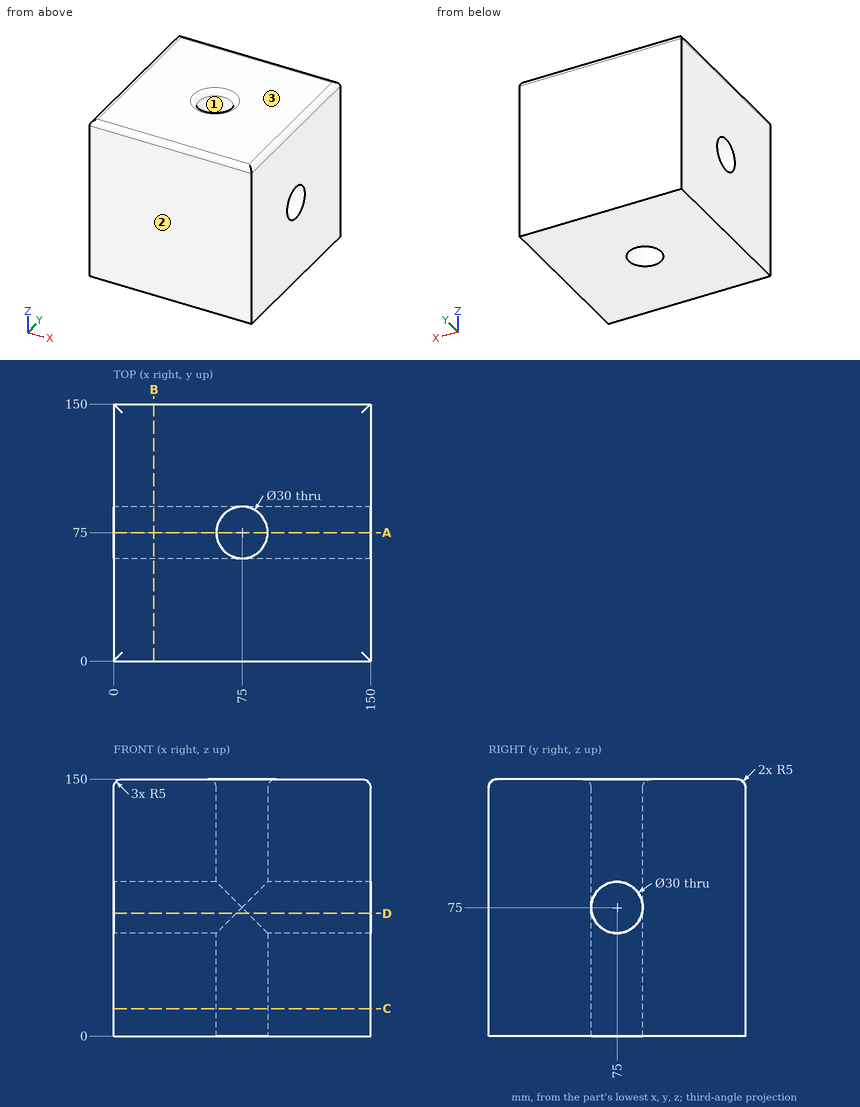
Here's the drawing with two shaded views (mm, measured from the low corner). I have some questions. Give positions to 0.01 mm unless a question says otherwise; leave off trailing zeros. Write each loop counter-clockwise with the first axis right and the second up, starting at its lowest first coordinate (ties: lowest second). Pieces come first, ordered by that corner, then holes. Notation, with made-up numbers: (-30.5, 43) - (-26.5, 43) arc R27 cw to (-26.5, 68) - close; hole circle Ø7 at (3, 25.25). An arc over 180 degrees is marked (long way). One line per item, written item: value. Start each with the question number.
Item 1: If we mould it in two halves opening along Y, with no side actions, what happens to the marked faces 1, 2 and 3? For each: +Y half, -Y half, draft (parallel to the pull), parting line (faces both ways), or undercut.
Item 2: Imagine slicing it at A-A, the plane y = 75. List the corners of the cut face in (x, z) for me.
Item 3: Imagine slicing it at D-D, the plane z = 71.5. List the corners of the cut face in (x, y) for me.
Item 4: Imagine slicing it at C-C, the plane z = 16. List the corners of the cut face in (x, y) for me, and give its area (3 significant figures).
Item 5: Please list where these lines run through material, in increasing order: line 1 (Y direction, x = 121, z = 75); line 2 (Y direction, x = 88.5, z = 33). Write a range as from..to.
Item 6: Imagine slicing it at B-B, the plane x = 23.5. List the corners of the cut face in (y, z) for me, and give its area (3 significant figures).
Geometry says:
1. face 1: undercut
1. face 2: -Y half
1. face 3: draft
2. outline: (0, 0) - (60, 0) - (60, 60) - (0, 60) - close; (0, 90) - (60, 90) - (60, 145) arc R5 ccw to (55, 150) - (5, 150) arc R5 ccw to (0, 145) - close; (90, 0) - (150, 0) - (150, 60) - (90, 60) - close; (90, 90) - (150, 90) - (150, 145) arc R5 ccw to (145, 150) - (95, 150) arc R5 ccw to (90, 145) - close
3. outline: (0, 0) - (150, 0) - (150, 60.41) - (78.5, 60.41) arc R15 cw to (71.5, 60.41) - (0, 60.41) - close; (0, 89.59) - (71.5, 89.59) arc R15 cw to (78.5, 89.59) - (150, 89.59) - (150, 150) - (0, 150) - close
4. outline: (0, 0) - (150, 0) - (150, 150) - (0, 150) - close; hole circle Ø30 at (75, 75)
4. area: 21,800 mm^2
5. line 1: 0..60, 90..150
5. line 2: 0..68.46, 81.54..150
6. outline: (0, 0) - (150, 0) - (150, 145) arc R5 ccw to (145, 150) - (5, 150) arc R5 ccw to (0, 145) - close; hole circle Ø30 at (75, 75)
6. area: 21,800 mm^2
